Design review of the part built by this model. Coordinates are the model's own, in mm. Face numbers are marked on the shaded views. A direction names the side the tool comes from. Coordinates: 2 decimals unless noted, no trailing zeros. Loops run counter-clockwise (first coordinate to the right, second up) from the corner with the lowest first, then second, coordinate; pieces in that order, holes last. Notation, with made-up numbers: (17, -34) -> (36, -34) arc R22 ccw to (36, -5) -> close; hole circle Ø10 at (-21.5, 81). An arc over 180 degrees is marked (long way). One line per item, written item: value. Start each with the question number.
1. Add section B-B on z = 12. Write out the cut boundary in (x, y).
2. Draft analysis for pull direction Y (two halves, no side actions). For the marked faces 1, 2 and 3, state which applies: pulls with the +Y half, pulls with the -Y half, needs draft (parallel to the pull), parting line crosses it, or undercut.
3. Add section D-D on y = 7. Write out the cut boundary in (x, z).
4. Insertion check: pin 1 (3 mm diameter, centred on y = 4.5, z = 13, fed in from -X); pin 2 (6 mm diameter, centred on x = -8, y = -0.5, fed in from -Z); pin 3 (1.8 mm diameter, centred on x = 4, y = 10, fed in from -Z). Each pin has a flat end and moves straight along its axis. Give the tip position at first contact, or say it passes through.
5. Machinability: for the marked faces 4, 5 and 6, which of the approach directions +Z, -Z, +X, -X, +Y, -Y give a long, thin tool a straight path to every point of the face, cutting with its end or side? Answer none if there is none.
6. Add section A-A on z = 3.25. Write out the cut boundary in (x, y), plus the area to 3 significant figures.
7. Add section C-C on x = 6. Write out the cut boundary in (y, z).
8. For probe 1 along Y at (x, z) = (4, 7.25); probe 2 along X at (y, z) = (-10, 8); probe 3 along Y at (x, z) = (0.5, 5.25), list the stretches that pass through material, from the lowest coordinate up.
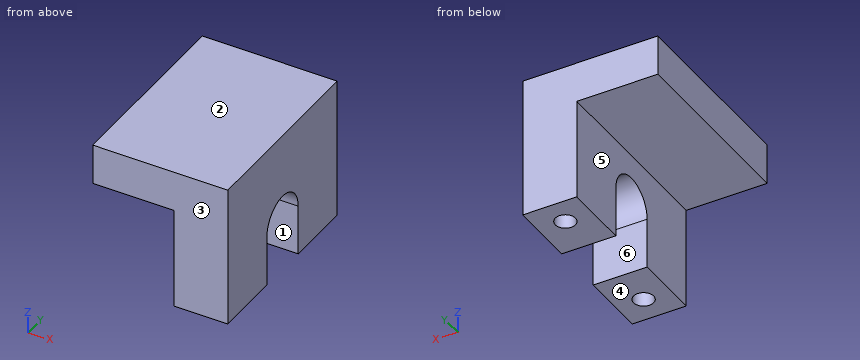
Autodesk Fusion 360 part; units mm, degrees
sketch "スケッチ1" plane through (0, 0, 0) normal (0, 0, 1) x (1, 0, 0)
  line L0 (0, -14) -> (8, -14)
  line L1 (8, -14) -> (8, 14)
  line L2 (8, 14) -> (0, 14)
  line L3 (0, 14) -> (0, -14)
  dimension "d1" = 8
  dimension "d2" = 28
extrude "押し出し1" add sketch "スケッチ1" along normal blind 15
sketch "スケッチ2" plane through (0, 0, 15) normal (0, 0, 1) x (-1, 0, 0)
  line L0 (0, -14) -> (0, 14)
  line L1 (0, 14) -> (-8, 14)
  line L2 (-8, 14) -> (-8, -14)
  line L3 (-8, -14) -> (0, -14)
  line L4 (12, -14) -> (-8, -14)
  line L5 (-8, -14) -> (-8, 14)
  line L6 (-8, 14) -> (12, 14)
  line L7 (12, 14) -> (12, -14)
  dimension "d5" = 20
extrude "押し出し2" add sketch "スケッチ2" along normal blind 6
sketch "スケッチ3" plane through (8, 0, 0) normal (1, 0, 0) x (0, 1, 0)
  line L0 (-14, 0) -> (14, 0)
  line L1 (14, 0) -> (14, 21)
  line L2 (14, 21) -> (-14, 21)
  line L3 (-14, 21) -> (-14, 0)
  line L4 (-4, 0) -> (4, 0)
  line L5 (4, 0) -> (4, 7.5)
  line L6 (4, 7.5) -> (-4, 7.5)
  line L7 (-4, 7.5) -> (-4, 0)
  circle A0 centre (0, 7.5) radius 4
  dimension "d8" = 8
  dimension "d9" = 7.5
extrude "押し出し3" cut sketch "スケッチ3" against normal through all contours L0 L4 L5 L7 A0 | L6 A0 | L6 A0
sketch "スケッチ4" plane through (0, 0, 0) normal (0, 0, -1) x (1, 0, 0)
  line L0 (0, 4) -> (8, 4)
  line L1 (8, 4) -> (8, 14)
  line L2 (8, 14) -> (0, 14)
  line L3 (0, 14) -> (0, 4)
  line L4 (4, 10) -> (4, -10)
  line L5 (8, -14) -> (0, -14)
  point P0 (4, 14)
  dimension "d11" = 4
  dimension "d12" = 4
hole "穴1" at (4, -10, 0) at (4, 10, 0) direction (0, 0, 1) diameter 3 depth 15 tip angle 118
thread "ねじ1"
Worked answers:
1. outline: (0, -14) -> (8, -14) -> (8, 14) -> (0, 14) -> close; hole circle Ø3 at (4, -10); hole circle Ø3 at (4, 10)
2. face 1: undercut
2. face 2: needs draft
2. face 3: pulls with the -Y half
3. outline: (-12, 15) -> (0, 15) -> (0, 0) -> (8, 0) -> (8, 21) -> (-12, 21) -> close
4. pin 1: stops at x = 0
4. pin 2: stops at z = 15
4. pin 3: stops at z = 15.36
5. face 4: -Z, +X, -X, +Y, -Y
5. face 5: -Z, -X, +Y, -Y
5. face 6: -Z, +X, -X
6. outline: (0, -14) -> (8, -14) -> (8, -4) -> (0, -4) -> close; (0, 4) -> (8, 4) -> (8, 14) -> (0, 14) -> close; hole circle Ø3 at (4, -10); hole circle Ø3 at (4, 10)
6. area: 146 mm²
7. outline: (-14, 0) -> (-4, 0) -> (-4, 7.5) arc R4 cw to (4, 7.5) -> (4, 0) -> (14, 0) -> (14, 21) -> (-14, 21) -> close
8. probe 1: y = -14 to -11.5, -8.5 to -4, 4 to 8.5, 11.5 to 14
8. probe 2: x = 0 to 2.5, 5.5 to 8
8. probe 3: y = -14 to -4, 4 to 14
